Geometry check sheet. Reference: the model listing, model coordinates, mm. Round coordinates to 2 decimals unless told otherwise and drop trailing zeros. Write each loop counter-clockwise with the first axis right and the second up, starting at its lowest first coordinate (ties: lowest second). Pieces come first, ordered by that corner, then holes. Notation, with made-up numbers: (60.25, -9) -> (106.25, -9) arc R22 cw to (106.25, 30) -> close; hole circle Ø10 at (18.25, 68). An arc over 180 degrees is marked (long way). Use a Markdown table: item, result.
```python
from build123d import *

# Parameters (mm, degrees)
SKETCH_W      = 20
SKETCH_H      = 20
PAD_DEPTH     = 20
SKETCH001_R   = 1.65
HOLE_DEPTH    = 10
HOLE_TIPS_R   = 1.65
SKETCH002_R   = 1.65
HOLE001_DEPTH = 20.001


with BuildPart() as part:
    # Sketch → Pad (new body)
    with BuildSketch(Plane.XY):
        with Locations((-75, 10)):
            Rectangle(SKETCH_W, SKETCH_H)
    extrude(amount=PAD_DEPTH)

    # Sketch001 (on Face1 of Pad) → Hole (cut)
    with BuildSketch(Plane.XZ):
        with Locations((-75, 10)):
            Circle(SKETCH001_R)
    extrude(amount=-HOLE_DEPTH, mode=Mode.SUBTRACT)

    # Hole tips → Hole tip 1 section 0
    with BuildSketch(Plane.XZ.offset(-10), mode=Mode.PRIVATE) as hole_tip_1_s0:
        with Locations((-75, 10)):
            Circle(HOLE_TIPS_R)
    loft([hole_tip_1_s0.sketch, Vertex(-75, 10.99142, 10)], mode=Mode.SUBTRACT)

    # Sketch002 (on Face4 of Hole) → Hole001 (cut, through all)
    with BuildSketch(Plane.XY.offset(20)):
        with Locations((-70, 10)):
            Circle(SKETCH002_R)
    extrude(amount=-HOLE001_DEPTH, mode=Mode.SUBTRACT)


solid = part.part
```
(1) Thickness scan on line 1 (Z direction, x = -75, y = 7.25); line 2 (Y direction, x = -71.5, z = 5.25). Record the ranges inside material, lowest first.
A:
| item | result |
|---|---|
| line 1 | z = 0 to 8.35, 11.65 to 20 |
| line 2 | y = 0 to 9.31, 10.69 to 20 |
(2) Section check A-A on z = 15.5. Record the cut outline in (x, y), plus the area to 3 significant figures.
A:
| item | result |
|---|---|
| outline | (-85, 0) -> (-65, 0) -> (-65, 20) -> (-85, 20) -> close; hole circle Ø3.3 at (-70, 10) |
| area | 391 mm2 |
(3) Release check for a two-part mould opening along X. For faces 1 (the face through (-85, 10, 10)), 2 (the face through (-76.65, 4.93, 10.07)), 3 (the face through (-65, 10, 10)), 4 (the face through (-75, 20, 10)) record: +X half, -X half, draft (parallel to the pull), parting line (faces both ways), or undercut.
A:
| item | result |
|---|---|
| face 1 | -X half |
| face 2 | undercut |
| face 3 | +X half |
| face 4 | draft |
(4) Section check B-B on y = 6.25. Record the cut outline in (x, z).
A:
| item | result |
|---|---|
| outline | (-85, 0) -> (-65, 0) -> (-65, 20) -> (-85, 20) -> close; hole circle Ø3.3 at (-75, 10) |
(5) Gauge pin test, flat end, axial feed: pin 1 Ø2.5 at (x, z) = (-75, 10) entering from -Y. Record the tip position at first contact, or that the pin passes through.
A:
| item | result |
|---|---|
| pin 1 | stops at y = 10.24 |
